Verification items for the finished model (mm, model axes). A direction names the side the tool comes from. Give positions to 0.01 mm unless a question says otherwise; leave off trailing zeros. Write each loop counter-clockwise with the first axis right and the second up, starting at its lowest first coordinate (ties: lowest second). Pieces come first, ordered by that corner, then holes. Notation, with made-up numbers: (64, 9) -> (70, 9) arc R26 cw to (70, 26) -> close; hole circle Ø3 at (16.5, 51.5). An arc over 180 degrees is marked (long way). Write item = value, one per line.
from build123d import *

# Parameters (mm, degrees)
SKETCH3_W           = 60
SKETCH3_H           = 100
BOSS_EXTRUDE1_DEPTH = 40
SHELL1_T            = -2
SKETCH2_R           = 3.5
SKETCH2_R_2         = 1.5
BOSS_EXTRUDE2_DEPTH = 2
CUT_EXTRUDE1_REACH  = 120.322
SKETCH4_W           = 60
SKETCH4_H           = 100
CUT_EXTRUDE2_REACH  = 118.636
SKETCH5_R           = 6
SKETCH6_W           = 6
SKETCH6_H           = 1
CUT_EXTRUDE3_DEPTH  = 2
BOSS_EXTRUDE3_DEPTH = 2
SKETCH7_W           = 8
SKETCH7_H           = 8
SKETCH7_R           = 1.5
BOSS_EXTRUDE4_DEPTH = 2


with BuildPart() as part:
    # Sketch3 → Boss-Extrude1 (new body)
    with BuildSketch(Plane(origin=(0, 0, 0), x_dir=(1, 0, 0), z_dir=(0, 1, 0))):
        with Locations((30, 50)):
            Rectangle(SKETCH3_W, SKETCH3_H)
    extrude(amount=BOSS_EXTRUDE1_DEPTH)

    # Shell1
    shell1_openings = [part.faces().sort_by_distance(p)[0] for p in [
        (30, 20, 0),
    ]]
    offset(amount=SHELL1_T, openings=shell1_openings, kind=Kind.INTERSECTION)

    # Sketch2 → Boss-Extrude2 (add)
    # profile 1 of 4: a face of its own
    with BuildSketch(Plane(origin=(0, 2, 0), x_dir=(1, 0, 0), z_dir=(0, 1, 0))):
        with Locations(Location((19.5, 17, 0), (0, 0, 90))):
            Circle(SKETCH2_R)
        with Locations(Location((19.5, 17, 0), (0, 0, 270))):
            Circle(SKETCH2_R_2, mode=Mode.SUBTRACT)
    # profile 2 of 4: a face of its own
    with BuildSketch(Plane(origin=(0, 2, 0), x_dir=(1, 0, 0), z_dir=(0, 1, 0))):
        with Locations(Location((40.5, 17, 0), (0, 0, 90))):
            Circle(SKETCH2_R)
        with Locations(Location((40.5, 17, 0), (0, 0, 270))):
            Circle(SKETCH2_R_2, mode=Mode.SUBTRACT)
    # profile 3 of 4: a face of its own
    with BuildSketch(Plane(origin=(0, 2, 0), x_dir=(1, 0, 0), z_dir=(0, 1, 0))):
        with Locations(Location((40.5, 45, 0), (0, 0, 90))):
            Circle(SKETCH2_R)
        with Locations(Location((40.5, 45, 0), (0, 0, 270))):
            Circle(SKETCH2_R_2, mode=Mode.SUBTRACT)
    # profile 4 of 4: a face of its own
    with BuildSketch(Plane(origin=(0, 2, 0), x_dir=(1, 0, 0), z_dir=(0, 1, 0))):
        with Locations(Location((19.5, 45, 0), (0, 0, 90))):
            Circle(SKETCH2_R)
        with Locations(Location((19.5, 45, 0), (0, 0, 270))):
            Circle(SKETCH2_R_2, mode=Mode.SUBTRACT)
    extrude(amount=BOSS_EXTRUDE2_DEPTH)

    # Sketch4 → Cut-Extrude1 (cut, up to next)
    with BuildSketch(Plane(origin=(0, 20, 0), x_dir=(1, 0, 0), z_dir=(0, 1, 0)), mode=Mode.PRIVATE) as cut_extrude1_sk1:
        with Locations((30, 50)):
            Rectangle(SKETCH4_W, SKETCH4_H)
    cut_extrude1_tool1 = extrude(cut_extrude1_sk1.sketch, amount=CUT_EXTRUDE1_REACH, mode=Mode.PRIVATE) & part.part
    add(cut_extrude1_tool1.solids().sort_by_distance((30, 20, -50))[0], mode=Mode.SUBTRACT)

    # Sketch5 → Cut-Extrude2 (cut, up to next)
    with BuildSketch(Plane.XY.offset(-98), mode=Mode.PRIVATE) as cut_extrude2_sk1:
        with Locations((30, 20)):
            Circle(SKETCH5_R)
    cut_extrude2_tool1 = extrude(cut_extrude2_sk1.sketch, amount=-CUT_EXTRUDE2_REACH, mode=Mode.PRIVATE) & part.part
    add(cut_extrude2_tool1.solids().sort_by_distance((30, 20, -98))[0], mode=Mode.SUBTRACT)

    # Sketch6 → Cut-Extrude3 (cut)
    with BuildSketch(Plane(origin=(0, 20, 0), x_dir=(1, 0, 0), z_dir=(0, 1, 0))):
        Polygon((60, 100), (36, 100), (36, 99), (59, 99), (59, 0), (60, 0), align=None)
        with Locations((33, 99.5)):
            Rectangle(SKETCH6_W, SKETCH6_H)
    extrude(amount=-CUT_EXTRUDE3_DEPTH, mode=Mode.SUBTRACT)

    # Sketch6_3 → Boss-Extrude3 (add)
    with BuildSketch(Plane(origin=(0, 20, 0), x_dir=(1, 0, 0), z_dir=(0, 1, 0))):
        Polygon((24, 99), (24, 100), (0, 100), (0, 0), (1, 0), (1, 99), align=None)
    extrude(amount=BOSS_EXTRUDE3_DEPTH)

    # Sketch7 → Boss-Extrude4 (add)
    with BuildSketch(Plane.XY):
        with Locations((64, 4)):
            Rectangle(SKETCH7_W, SKETCH7_H)
        with Locations((64, 4)):
            Circle(SKETCH7_R, mode=Mode.SUBTRACT)
    extrude(amount=-BOSS_EXTRUDE4_DEPTH)


solid = part.part
Item 1: Sectioned sample at C-C on y = 15. Record the cut outline in (x, z), then the cut area to 3 significant figures.
Response values:
outline = (0, -100) -> (26.68, -100) -> (26.68, -98) -> (2, -98) -> (2, 0) -> (0, 0) -> close; (33.32, -100) -> (60, -100) -> (60, 0) -> (58, 0) -> (58, -98) -> (33.32, -98) -> close
area = 499 mm^2
Item 2: Sectioned sample at A-A on x = 64. Record the cut outline in (y, z), then the cut area to 3 significant figures.
Response values:
outline = (0, -2) -> (2.5, -2) -> (2.5, 0) -> (0, 0) -> close; (5.5, -2) -> (8, -2) -> (8, 0) -> (5.5, 0) -> close
area = 10.0 mm^2
Item 3: Set-up check for faces 1 (the cylindrical face through (65.43, 4.45, -0.99)), 2 (the flat face through (40, 4, -47)), 3 (the flat face through (40, 2, -45)), 4 (the flat face through (12, 21, -99)), 5 (the flat face through (59, 19, -50)): record each of +Z, -Z, +X, -X, +Y, -Y from which the full face is reachable in a straight line by a thin tool's end or side.
Response values:
face_1 = +Z, -Z
face_2 = +Z, +Y
face_3 = +Y
face_4 = +Z, +X, +Y
face_5 = +Z, -Z, +X, +Y
Item 4: Sectioned sample at D-D on x = 54. Record the cut outline in (y, z).
Response values:
outline = (0, -100) -> (18, -100) -> (18, -99) -> (20, -99) -> (20, -98) -> (2, -98) -> (2, 0) -> (0, 0) -> close
Item 5: Go/stop test with flat-tipped pins: P1, Ø2, axis at x = 41.5, z = -18, coming from the +Y side; P2, Ø3, axis at y = 5.5, z = -66.5, coming from the +X side; P3, Ø3.5, axis at x = 19.5, z = -17, coming from the -Y side; P4, Ø7, axis at x = 42, z = -28.5, coming from the +Y side. Record where each tip stops, or that it passes through.
Response values:
P1 = 4
P2 = 60
P3 = 0
P4 = 2
Item 6: Mould release check, pull along Z, two halves, no side actions. Record for faces 6 (the flat face through (62, 4, -2)), 7 (the cylindrical face through (19.346, 2.986, -41.503)), 8 (the flat face through (19, 4, -19)), 9 (the cylindrical face through (20.51, 2.99, -18.11)): +Z half, -Z half, draft (parallel to the pull), parting line (faces both ways), or undercut.
Response values:
face_6 = -Z half
face_7 = undercut
face_8 = draft
face_9 = undercut
Item 7: Material ranges on line 1 (X direction, y = 3.4, z = -45); line 2 (X direction, y = 12.25, z = -37.5); line 3 (Y direction, x = 40.5, z = -92.5), recorded low to high.
Response values:
line_1 = 0 to 2, 16 to 18, 21 to 23, 37 to 39, 42 to 44, 58 to 60
line_2 = 0 to 2, 58 to 60
line_3 = 0 to 2
Item 8: Sectioned sample at B-B on z = -45. Record the cut outline in (x, y).
Response values:
outline = (0, 0) -> (60, 0) -> (60, 18) -> (59, 18) -> (59, 20) -> (58, 20) -> (58, 2) -> (44, 2) -> (44, 4) -> (42, 4) -> (42, 2) -> (39, 2) -> (39, 4) -> (37, 4) -> (37, 2) -> (23, 2) -> (23, 4) -> (21, 4) -> (21, 2) -> (18, 2) -> (18, 4) -> (16, 4) -> (16, 2) -> (2, 2) -> (2, 20) -> (1, 20) -> (1, 22) -> (0, 22) -> close
